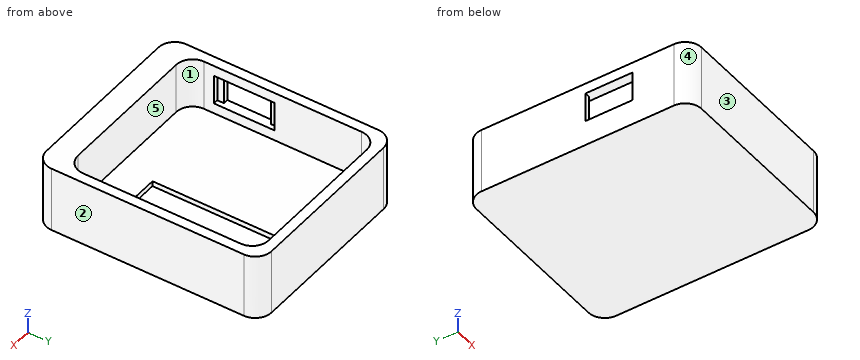
```python
from build123d import *

# Parameters (mm, degrees)
F0_W      = 47.5
F0_H      = 27.5
F0_W_2    = 37.5
F0_H_2    = 17.5
F1_DEPTH  = 4.6
F2_DEPTH  = 1.6
F7_ANGLE  = 90
F8_W      = 17.5
F8_H      = 37.5
F9_DEPTH  = 4.6
F10_DEPTH = 20
F11_W     = 14.4
F11_H     = 9
F12_DEPTH = 3
F13_W     = 2
F13_H     = 9
F14_DEPTH = 1.5


with BuildPart() as f1:
    # F0 (on Top) → F1 (new body)
    with BuildSketch(Plane.XY):
        Rectangle(F0_W, F0_H)
        Rectangle(F0_W_2, F0_H_2, mode=Mode.SUBTRACT)
        Rectangle(F0_W_2, F0_H_2)
    extrude(amount=F1_DEPTH)

    # F0 (on Top) → F2 (cut)
    with BuildSketch(Plane.XY):
        Rectangle(F0_W_2, F0_H_2)
    extrude(amount=F2_DEPTH, mode=Mode.SUBTRACT)


with BuildPart() as f4_1:
    # F4: instance of F1
    add(f1.part.mirror(Plane.XY.offset(2.3)))


with BuildPart() as f4_1_1:
    # F7: moved
    add(f4_1.part.rotate(Axis((0, 0, 16.2241663784), (0, 0, 1)), F7_ANGLE))

    # F8 (on Top) → F9 (join, through all)
    with BuildSketch(Plane.XY):
        with BuildLine():
            Line((11.75, 31.75), (-37.25, 31.75))
            ThreePointArc((-37.25, 31.75), (-40.7855339059, 30.2855339059), (-42.25, 26.75))
            Line((-42.25, 26.75), (-42.25, -31.75))
            ThreePointArc((-42.25, -31.75), (-40.7855339059, -35.2855339059), (-37.25, -36.75))
            Line((-37.25, -36.75), (11.75, -36.75))
            ThreePointArc((11.75, -36.75), (15.2855339059, -35.2855339059), (16.75, -31.75))
            Line((16.75, -31.75), (16.75, 26.75))
            ThreePointArc((16.75, 26.75), (15.2855339059, 30.2855339059), (11.75, 31.75))
        make_face()
        with BuildLine():
            ThreePointArc((-34.25, -29.25), (-37.7855339059, -27.7855339059), (-39.25, -24.25))
            Line((-39.25, -24.25), (-39.25, 23.75))
            ThreePointArc((-39.25, 23.75), (-37.7855339059, 27.2855339059), (-34.25, 28.75))
            Line((-34.25, 28.75), (8.75, 28.75))
            ThreePointArc((8.75, 28.75), (12.2855339059, 27.2855339059), (13.75, 23.75))
            Line((13.75, 23.75), (13.75, -24.25))
            ThreePointArc((13.75, -24.25), (12.2855339059, -27.7855339059), (8.75, -29.25))
            Line((8.75, -29.25), (-34.25, -29.25))
        make_face(mode=Mode.SUBTRACT)
        with BuildLine():
            Line((-39.25, 23.75), (-39.25, -24.25))
            ThreePointArc((-39.25, -24.25), (-37.7855339059, -27.7855339059), (-34.25, -29.25))
            Line((-34.25, -29.25), (8.75, -29.25))
            ThreePointArc((8.75, -29.25), (12.2855339059, -27.7855339059), (13.75, -24.25))
            Line((13.75, -24.25), (13.75, 23.75))
            ThreePointArc((13.75, 23.75), (12.2855339059, 27.2855339059), (8.75, 28.75))
            Line((8.75, 28.75), (-34.25, 28.75))
            ThreePointArc((-34.25, 28.75), (-37.7855339059, 27.2855339059), (-39.25, 23.75))
        make_face()
        Rectangle(F8_W, F8_H, mode=Mode.SUBTRACT)
    extrude(amount=F9_DEPTH)

    # F8 (on Top) → F10 (join)
    with BuildSketch(Plane.XY):
        with BuildLine():
            Line((11.75, 31.75), (-37.25, 31.75))
            ThreePointArc((-37.25, 31.75), (-40.7855339059, 30.2855339059), (-42.25, 26.75))
            Line((-42.25, 26.75), (-42.25, -31.75))
            ThreePointArc((-42.25, -31.75), (-40.7855339059, -35.2855339059), (-37.25, -36.75))
            Line((-37.25, -36.75), (11.75, -36.75))
            ThreePointArc((11.75, -36.75), (15.2855339059, -35.2855339059), (16.75, -31.75))
            Line((16.75, -31.75), (16.75, 26.75))
            ThreePointArc((16.75, 26.75), (15.2855339059, 30.2855339059), (11.75, 31.75))
        make_face()
        with BuildLine():
            ThreePointArc((-34.25, -29.25), (-37.7855339059, -27.7855339059), (-39.25, -24.25))
            Line((-39.25, -24.25), (-39.25, 23.75))
            ThreePointArc((-39.25, 23.75), (-37.7855339059, 27.2855339059), (-34.25, 28.75))
            Line((-34.25, 28.75), (8.75, 28.75))
            ThreePointArc((8.75, 28.75), (12.2855339059, 27.2855339059), (13.75, 23.75))
            Line((13.75, 23.75), (13.75, -24.25))
            ThreePointArc((13.75, -24.25), (12.2855339059, -27.7855339059), (8.75, -29.25))
            Line((8.75, -29.25), (-34.25, -29.25))
        make_face(mode=Mode.SUBTRACT)
    extrude(amount=F10_DEPTH)

    # F11 (on face) → F12 (cut, through all)
    with BuildSketch(Plane(origin=(-42.25, 0, 0), x_dir=(0, -1, 0), z_dir=(-1, 0, 0))):
        with Locations((12.05, 12.3)):
            Rectangle(F11_W, F11_H)
    extrude(amount=-F12_DEPTH, mode=Mode.SUBTRACT)

    # F13 (on face) → F14 (cut)
    with BuildSketch(Plane.YZ.offset(-39.25)):
        with Locations((-20.25, 12.3)):
            Rectangle(F13_W, F13_H)
        with Locations((-3.85, 12.3)):
            Rectangle(F13_W, F13_H)
    extrude(amount=-F14_DEPTH, mode=Mode.SUBTRACT)


solid = f4_1_1.part
```
Can you work these out from the model? Positions are in its coordinate system, mm. Face numbers are marked on the shaded views. A direction names the side the tool comes from. Coordinates: 2 decimals unless noted, no trailing zeros. Order: outer loops, then holes, each group sorted by start corner. A loop starts at its lowest first (then second) coordinate and runs counter-clockwise, first axis right, second up.
1. If we section it at D-D (x = 4.5): Please give me the cut outline in (y, z), then the cut area to 3 significant figures.
2. I'm going to push flat-ended pins straight in: pin 1 (0.8 mm diameter, centred on x = -40.5, z = 12.5, fed in from +Y); pin 2 (0.8 mm diameter, centred on x = -41.5, z = 13, fed in from +Y); pin 3 (4 mm diameter, centred on x = -8, y = 18, fed in from +Z). Where does each tip first touch, or does it pass through?
3. If we section it at B-B (y = -18): Please give me the cut outline in (x, z).
4. If we section it at C-C (z = 11.25): Please give me the cut outline in (x, y), then the cut area to 3 significant figures.
5. Thinking about a two-plate mould opening in X: for the marked faces 1, 2 and 3, which applies, +X half, -X half, draft (parallel to the pull), parting line (faces both ways), or undercut?
6. I need wall thicknesses on line 1 (X direction, y = 2, z = 7.75); line 2 (Y direction, x = -21, z = 13.25); line 3 (Y direction, x = -34.5, z = 13). Which ranges of each line are inside material? Lowest first, please.
7. If we section it at A-A (z = 6.25): Please give me the cut outline in (x, y).
8. For the marked faces 4 and 5, which set-ups out of +Z, -Z, +X, -X, +Y, -Y let a thin tool reach every point of the face, with its end or its side?
Entries:
1. outline: (-36.75, 0) - (31.75, 0) - (31.75, 20) - (28.75, 20) - (28.75, 4.6) - (18.75, 4.6) - (18.75, 3) - (-18.75, 3) - (-18.75, 4.6) - (-29.25, 4.6) - (-29.25, 20) - (-36.75, 20) - close
1. area: 417 mm2
2. pin 1: stops at y = 30.86
2. pin 2: stops at y = 29.94
2. pin 3: stops at z = 4.6
3. outline: (-42.25, 0) - (16.75, 0) - (16.75, 20) - (13.75, 20) - (13.75, 4.6) - (8.75, 4.6) - (8.75, 3) - (-8.75, 3) - (-8.75, 4.6) - (-39.25, 4.6) - (-39.25, 7.8) - (-42.25, 7.8) - close; (-42.25, 16.8) - (-39.25, 16.8) - (-39.25, 20) - (-42.25, 20) - close
4. outline: (-42.25, -31.75) arc R5 ccw to (-37.25, -36.75) - (11.75, -36.75) arc R5 ccw to (16.75, -31.75) - (16.75, 26.75) arc R5 ccw to (11.75, 31.75) - (-37.25, 31.75) arc R5 ccw to (-42.25, 26.75) - (-42.25, -4.85) - (-40.75, -4.85) - (-40.75, -2.85) - (-39.25, -2.85) - (-39.25, 23.75) arc R5 cw to (-34.25, 28.75) - (8.75, 28.75) arc R5 cw to (13.75, 23.75) - (13.75, -24.25) arc R5 cw to (8.75, -29.25) - (-34.25, -29.25) arc R5 cw to (-39.25, -24.25) - (-39.25, -21.25) - (-40.75, -21.25) - (-40.75, -19.25) - (-42.25, -19.25) - close
4. area: 918 mm2
5. face 1: undercut
5. face 2: +X half
5. face 3: draft
6. line 1: x = -42.25 to -39.25, 13.75 to 16.75
6. line 2: y = -36.75 to -29.25, 28.75 to 31.75
6. line 3: y = -36.75 to -29.24, 28.74 to 31.75
7. outline: (-42.25, -31.75) arc R5 ccw to (-37.25, -36.75) - (11.75, -36.75) arc R5 ccw to (16.75, -31.75) - (16.75, 26.75) arc R5 ccw to (11.75, 31.75) - (-37.25, 31.75) arc R5 ccw to (-42.25, 26.75) - close; hole (-39.25, -24.25) arc R5 ccw to (-34.25, -29.25) - (8.75, -29.25) arc R5 ccw to (13.75, -24.25) - (13.75, 23.75) arc R5 ccw to (8.75, 28.75) - (-34.25, 28.75) arc R5 ccw to (-39.25, 23.75) - close
8. face 4: +Z, -Z, -X, -Y
8. face 5: +Z
